The model under review builds one solid part; all positions refer to its coordinate system, in mm. Give positions to 0.01 mm unless a question says otherwise; leave off trailing zeros. Write each loop counter-clockwise with the first axis right and the second up, starting at its lowest first coordinate (ties: lowest second). Pieces come first, ordered by that corner, then holes. Notation, with made-up numbers: M 81.25,-18.75 L 109.25,-18.75 A21 ccw 109.25,17.25 Z; hole C -30.75,53 d3. An arc over 180 degrees is marked long. Write item = value, one per line. Start each with the question number.
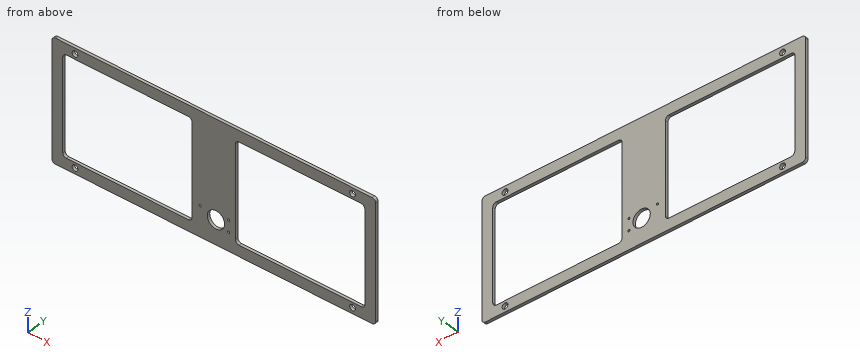
```python
from build123d import *

# Parameters (mm, degrees)
SKETCH1_W             = 200
SKETCH1_H             = 82.6
BASE_FLANGE1_DEPTH    = 2
SKETCH6_R             = 2
CUT_EXTRUDE1_DEPTH    = 148.587569056
SKETCH7_W             = 77.5
SKETCH7_H             = 67.6
CUT_EXTRUDE2_DEPTH    = 148.587569056
SKETCH8_W             = 82.6
SKETCH8_H             = 2
BOSS_EXTRUDE1_DEPTH   = 12
SKETCH9_W             = 82.6
SKETCH9_H             = 2
BOSS_EXTRUDE2_DEPTH   = 12
SKETCH10_W            = 12
SKETCH10_H            = 67.6
CUT_EXTRUDE3_DEPTH    = 159.943577694
FILLET1_R             = 2.5
SKETCH11_R            = 6
CUT_EXTRUDE4_DEPTH    = 159.943577694
F_1_5MM_DOWEL_HOLE1_D = 1.5


# Sheet-metal steps are written as plain solids
with BuildPart() as part:
    # Sketch1 → Base-Flange1 (new body)
    with BuildSketch(Plane(origin=(0, 0, 0), x_dir=(1, 0, 0), z_dir=(0, 1, 0))):
        with Locations((39.040431267, 8.155525606)):
            Rectangle(SKETCH1_W, SKETCH1_H)
    extrude(amount=-BASE_FLANGE1_DEPTH)

    # Sketch6 → Cut-Extrude1 (cut, through all)
    with BuildSketch(Plane(origin=(0, 0, 0), x_dir=(1, 0, 0), z_dir=(0, 1, 0))):
        with Locations(Location((-56.959568733, 45.455525606, 0), (0, 0, 270))):
            Circle(SKETCH6_R)
        with Locations(Location((-56.959568733, -29.144474394, 0), (0, 0, 270))):
            Circle(SKETCH6_R)
        with Locations(Location((135.040431267, -29.144474394, 0), (0, 0, 270))):
            Circle(SKETCH6_R)
        with Locations(Location((135.040431267, 45.455525606, 0), (0, 0, 270))):
            Circle(SKETCH6_R)
    extrude(amount=-CUT_EXTRUDE1_DEPTH, mode=Mode.SUBTRACT)

    # Sketch7 → Cut-Extrude2 (cut, through all)
    with BuildSketch(Plane(origin=(0, 0, 0), x_dir=(1, 0, 0), z_dir=(0, 1, 0))):
        with Locations((-14.709568733, 8.155525606)):
            Rectangle(SKETCH7_W, SKETCH7_H)
        with Locations((92.790431267, 8.155525606)):
            Rectangle(SKETCH7_W, SKETCH7_H)
    extrude(amount=-CUT_EXTRUDE2_DEPTH, mode=Mode.SUBTRACT)

    # Sketch8 → Boss-Extrude1 (add)
    with BuildSketch(Plane.ZY.offset(60.959568733)):
        with Locations((-8.155525606, -1)):
            Rectangle(SKETCH8_W, SKETCH8_H)
    extrude(amount=BOSS_EXTRUDE1_DEPTH)

    # Sketch9 → Boss-Extrude2 (add)
    with BuildSketch(Plane(origin=(139.040431267, 0, 0), x_dir=(0, 0, -1), z_dir=(1, 0, 0))):
        with Locations((8.155525606, -1)):
            Rectangle(SKETCH9_W, SKETCH9_H)
    extrude(amount=BOSS_EXTRUDE2_DEPTH)

    # Sketch10 → Cut-Extrude3 (cut, through all)
    with BuildSketch(Plane(origin=(0, 0, 0), x_dir=(1, 0, 0), z_dir=(0, 1, 0))):
        with Locations((-59.459568733, 8.155525606)):
            Rectangle(SKETCH10_W, SKETCH10_H)
        with Locations((137.540431267, 8.155525606)):
            Rectangle(SKETCH10_W, SKETCH10_H)
    extrude(amount=-CUT_EXTRUDE3_DEPTH, mode=Mode.SUBTRACT)

    # Fillet1
    fillet1_edges = [part.edges().sort_by_distance(p)[0] for p in [
        (-65.459568733, -1, 25.644474394),
        (-65.459568733, -1, -41.955525606),
        (143.540431267, -1, -41.955525606),
        (143.540431267, -1, 25.644474394),
        (24.040431267, -1, -41.955525606),
        (24.040431267, -1, 25.644474394),
        (54.040431267, -1, 25.644474394),
        (54.040431267, -1, -41.955525606),
        (-72.959568733, -1, -49.455525606),
        (-72.959568733, -1, 33.144474394),
        (151.040431267, -1, -49.455525606),
        (151.040431267, -1, 33.144474394),
    ]]
    fillet(fillet1_edges, radius=FILLET1_R)

    # Sketch11 → Cut-Extrude4 (cut, through all)
    with BuildSketch(Plane(origin=(0, 0, 0), x_dir=(1, 0, 0), z_dir=(0, 1, 0))):
        with Locations(Location((40.540479107, 32.955525606, 0), (0, 0, 270))):
            Circle(SKETCH11_R)
    extrude(amount=-CUT_EXTRUDE4_DEPTH, mode=Mode.SUBTRACT)

    # Ø1.5mm Dowel Hole1 (through all)
    with Locations(Plane(origin=(0, 0, 0), x_dir=(1, 0, 0), z_dir=(0, 1, 0))):
        with Locations((49.340479107, 36.955525606), (49.340479107, 28.955525606), (29.540479107, 28.955525606)):
            Hole(F_1_5MM_DOWEL_HOLE1_D / 2)


solid = part.part
```
Item 1: Clearance check with flat-ended pins moving along their axes: P1, Ø14, axis at x = 40.54, z = -32.96, coming from the -Y side; P2, Ø3.5, axis at x = -56.96, z = -45.46, coming from the +Y side. State where each tip first meets the part, or that it passes through.
Item 2: To check wall thickness, follow probe 1 along X at (y, z) = (-1.5, -2); probe 2 along Z at (x, y) = (56.5, -0.95); probe 3 along X at (y, z) = (-1.25, -40). State the ranges of each line that lie inside material, in increasing order. Write a range as [from, to].
Item 3: We need section B-B, the plane x = 126. Write out the cut boundary in (y, z), and give its area (3 significant figures).
Item 4: We need section C-C, the plane y = -0.75. Give the number of separate pieces and of enclosed holes in the cut face, and give its area (3 significant figures).
Item 5: We need section A-A, the plane z = 2. Write out the cut boundary in (x, y).
Worked out:
q1.P1 = -2
q1.P2 = through
q2.probe_1 = [-72.96, -65.46], [24.04, 54.04], [143.54, 151.04]
q2.probe_2 = [-49.46, -41.96], [25.64, 33.14]
q2.probe_3 = [-72.96, -65.4], [23.98, 54.1], [143.48, 151.04]
q3.outline = M -2,-49.46 L 0,-49.46 L 0,-41.96 L -2,-41.96 Z; M -2,25.64 L 0,25.64 L 0,33.14 L -2,33.14 Z
q3.area = 30.0 mm²
q4.separate_pieces = 1
q4.enclosed_holes = 10
q4.area = 6,240 mm²
q5.outline = M -72.96,-2 L -65.46,-2 L -65.46,0 L -72.96,0 Z; M 24.04,-2 L 54.04,-2 L 54.04,0 L 24.04,0 Z; M 143.54,-2 L 151.04,-2 L 151.04,0 L 143.54,0 Z
